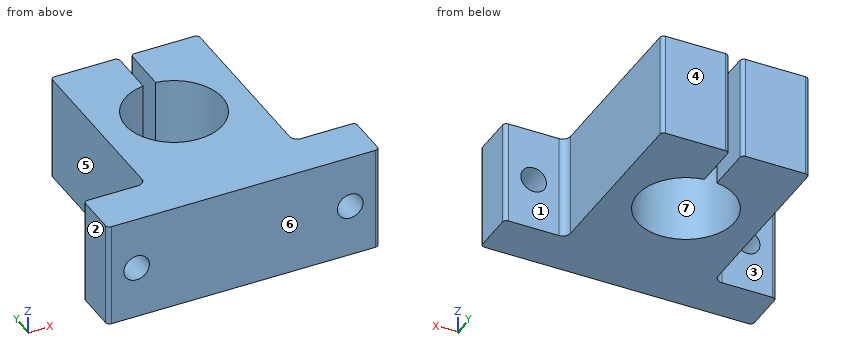
```python
from build123d import *

# Parameters (mm, degrees)
BOSS_EXTRUDE1_DEPTH = 27
SKETCH2_R           = 3.3
CUT_EXTRUDE1_DEPTH  = 66.253352404


with BuildPart() as part:
    # Sketch1 → Boss-Extrude1 (new body)
    with BuildSketch(Plane.XY):
        with BuildLine():
            Line((-35, -34), (-35, -24))
            ThreePointArc((-35, -24), (-34.707106781, -23.292893219), (-34, -23))
            Line((-34, -23), (-21, -23))
            ThreePointArc((-21, -23), (-19.585786438, -22.414213562), (-19, -21))
            Line((-19, -21), (-19, 24))
            ThreePointArc((-19, 24), (-18.707106781, 24.707106781), (-18, 25))
            Line((-18, 25), (-2.6, 25))
            ThreePointArc((-2.6, 25), (-1.892893219, 24.707106781), (-1.6, 24))
            Line((-1.6, 24), (-1.6, 12.397177098))
            ThreePointArc((-1.6, 12.397177098), (0, -12.5), (1.6, 12.397177098))
            Line((1.6, 12.397177098), (1.6, 24))
            ThreePointArc((1.6, 24), (1.892893219, 24.707106781), (2.6, 25))
            Line((2.6, 25), (18, 25))
            ThreePointArc((18, 25), (18.707106781, 24.707106781), (19, 24))
            Line((19, 24), (19, -21))
            ThreePointArc((19, -21), (19.585786438, -22.414213562), (21, -23))
            Line((21, -23), (34, -23))
            ThreePointArc((34, -23), (34.707106781, -23.292893219), (35, -24))
            Line((35, -24), (35, -34))
            ThreePointArc((35, -34), (34.707106781, -34.707106781), (34, -35))
            Line((34, -35), (-34, -35))
            ThreePointArc((-34, -35), (-34.707106781, -34.707106781), (-35, -34))
        make_face()
    extrude(amount=BOSS_EXTRUDE1_DEPTH)

    # Sketch2 → Cut-Extrude1 (cut, through all)
    with BuildSketch(Plane(origin=(0, -23, 0), x_dir=(1, 0, 0), z_dir=(0, 1, 0))):
        with Locations(Location((-27.5, -13.5, 0), (0, 0, 270))):
            Circle(SKETCH2_R)
    cut_extrude1 = extrude(amount=-CUT_EXTRUDE1_DEPTH, mode=Mode.SUBTRACT)

    # Mirror1: Cut-Extrude1 across plane
    add(cut_extrude1.mirror(Plane(origin=(0, 0, 0), x_dir=(0, 0, 1), z_dir=(1, 0, 0))), mode=Mode.SUBTRACT)


solid = part.part
```
Build history of the part. All positions in model axes, mm. Face numbers are marked on the shaded views. A direction names the side the tool comes from. Give positions to 0.01 mm unless a question says otherwise; leave off trailing zeros. Order: outer loops, then holes, each group sorted by start corner. A loop starts at its lowest first (then second) coordinate and runs counter-clockwise, first axis right, second up. Notation, with made-up numbers: M -21.5,75.5 L 12.5,75.5 A9 ccw 12.5,90.5 Z; hole C -14,-7 d4. An arc over 180 degrees is marked long. Write item = value, one per line. Start each with the question number.
(1) Slice it at D-D on z = 9. Write the cut outline in (x, y), plus the area to 3 significant figures.
(2) Probe L1, parallel to X at y = -30.75, z = 13.5; L2, parallel to X at y = 15.5, z = 13.75; L3, parallel to Y at x = 0, z = 18. List the from-to ranges inside material, lowest first. Write a range as [from, to].
(3) Two-plate mould, pull along Y, no slides. Class the marked faces 4, 5, 6 and 7: released by +Y, released by -Y, zero draft, split by the parting line, or undercut.
(4) Slice it at A-A on y = 0. Write the cut outline in (x, z), plus the area to 3 significant figures.
(5) Slice it at B-B on z = 13.5. State how many separate pieces and enclosed holes the cut face has, plus the area to 3 significant figures.
(6) Which spindle directions (+Z, -Z, +X, -X, +Y, -Y) get a long thin tool onto all of the face, cutting with end or side? Do the marked faces 1, 2 and 3. Say none if no direction does.
(7) Slice it at C-C on x = 6. Write the cut outline in (y, z).
(8) Pin check, flat tips, straight feed: pin 1 Ø13 at (y, z) = (17.5, 8) entering from -X; pin 2 Ø1.5 at (x, z) = (-1.5, 3) entering from +Y; pin 3 Ø14.5 at (x, z) = (28.5, 19) entering from +Y. Stop position of each tip, or through.
Responses:
q1.outline = M -35,-34 A1 ccw -34,-35 L 34,-35 A1 ccw 35,-34 L 35,-24 A1 ccw 34,-23 L 21,-23 A2 cw 19,-21 L 19,24 A1 ccw 18,25 L 2.6,25 A1 ccw 1.6,24 L 1.6,12.4 A12.5 cw long -1.6,12.4 L -1.6,24 A1 ccw -2.6,25 L -18,25 A1 ccw -19,24 L -19,-21 A2 cw -21,-23 L -34,-23 A1 ccw -35,-24 Z
q1.area = 2,130 mm2
q2.L1 = [-35, -30.8], [-24.2, 24.2], [30.8, 35]
q2.L2 = [-19, -1.6], [1.6, 19]
q2.L3 = [-35, -12.5]
q3.face_4 = released by +Y
q3.face_5 = zero draft
q3.face_6 = released by -Y
q3.face_7 = undercut
q4.outline = M -19,0 L -12.5,0 L -12.5,27 L -19,27 Z; M 12.5,0 L 19,0 L 19,27 L 12.5,27 Z
q4.area = 351 mm2
q5.separate_pieces = 3
q5.enclosed_holes = 0
q5.area = 1,970 mm2
q6.face_1 = +Z, -Z, +X, +Y
q6.face_2 = +Z, -Z, -X, +Y, -Y
q6.face_3 = +Z, -Z, -X, +Y
q7.outline = M -35,0 L -10.97,0 L -10.97,27 L -35,27 Z; M 10.97,0 L 25,0 L 25,27 L 10.97,27 Z
q8.pin_1 = -19
q8.pin_2 = 24.94
q8.pin_3 = -23
